Source: three-view drawing plus pictorial views. Frame: mm from the lowest corner of the part. A direction names the side the tool comes from. Give positions to 0.01 mm unless a question says otherwise; leave off trailing zeros. Order: outer loops, then holes, each group sorted by start corner. A loop starts at its lowest first (then second) coordinate and runs counter-clockwise, first axis right, second up.
1) Material intervals for line 1 (Y direction, x = 5, z = 14) (3 decimals); line 2 (Y direction, x = 5, z = 7.75); line 3 (Z direction, x = 3, y = 6.75), sorted ascending.
2) Access query for the marked faces 1 and 2. Directions: +Z, -Z, +X, -X, +Y, -Y. A direction counts if a zero-diameter tool reaches every point of the face in a straight line with its end or side. Return the directions, or none.
3) Draft query along X for the marked faces 3, 4 and 5. Return one class per face: released by +X, released by -X, zero draft, split by the parting line, or undercut.
4) Section C-C, the plane z = 14.5. Return loops of the section in (x, y) (3 decimals).
5) Section A-A, the plane y = 5. Return loops of the section in (x, z) (3 decimals).
6) Section D-D, the plane z = 4. Return loops of the section in (x, y).
7) First-contact query: P1, Ø4, axis at x = 3.5, z = 3, coming from the +Y side; P2, Ø2, axis at y = 7.5, z = 13, coming from the -X side; P3, Ø3.5, axis at x = 5, y = 5, coming from the +Z side; P4, Ø2, axis at x = 3, z = 15, coming from the +Y side. Flat tips, straight axial feed; report the tip coordinate or a pass-through.
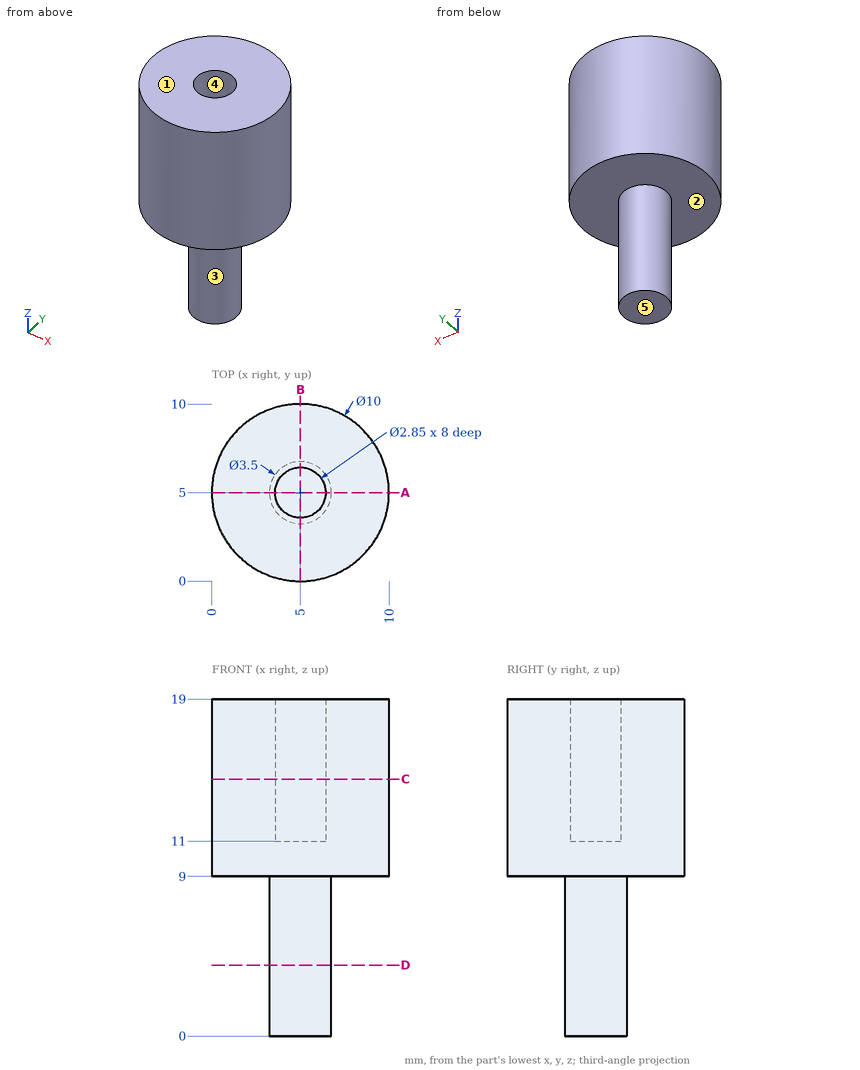
From the geometry:
1. line 1: y = 0 to 3.575, 6.425 to 10
1. line 2: y = 3.25 to 6.75
1. line 3: z = 9 to 19
2. face 1: +Z, +X, -X, +Y, -Y
2. face 2: -Z
3. face 3: split by the parting line
3. face 4: undercut
3. face 5: zero draft
4. outline: circle Ø10 at (5, 5); hole circle Ø2.85 at (5, 5)
5. outline: (0, 9) - (3.25, 9) - (3.25, 0) - (6.75, 0) - (6.75, 9) - (10, 9) - (10, 19) - (6.425, 19) - (6.425, 11) - (3.575, 11) - (3.575, 19) - (0, 19) - close
6. outline: circle Ø3.5 at (5, 5)
7. P1: stops at y = 6.75
7. P2: stops at x = 0.23
7. P3: stops at z = 19
7. P4: stops at y = 9.9
